Design review of the part built by this model. Coordinates are the model's own, in mm. A direction names the side the tool comes from. Coordinates: 2 decimals unless noted, no trailing zeros. Write each loop counter-clockwise with the first axis right and the second up, starting at its lowest first coordinate (ties: lowest second). Pieces come first, ordered by that corner, then holes.
Q1. Take a section at B-B (z = 0). Give the boundary of the cut face in (x, y), and give its area (3 significant figures).
Q2. For probe 1 along X at (y, z) = (1, 0); probe 2 along X at (y, z) = (-2.5, -5); probe 3 along Y at (x, z) = (6.5, 5.5), list the stretches that pass through material, from the lowest coordinate up.
Q3. Machinability: for faces 1 (the flat face through (-11.9, -1, -23.4)), 2 (the cylindrical face through (25.297, -0.507, -25.359)), 3 (the flat face through (-16, 0, 20)), which of the approach directions +Z, -Z, +X, -X, +Y, -Y give a long, thin tool a straight path to every point of the face, cutting with its end or side? Answer none if there is none.
Q4. Take a section at C-C (y = -23). Give the boundary of the cut face in (x, z).
Q5. Insertion check: pin 1 (6 mm diameter, centred on y = -26.5, z = 6.5, fed in from -X); pin 2 (2 mm diameter, centred on y = -2.5, z = 7, fed in from -X); pin 3 (1.5 mm diameter, centred on x = 4.5, y = -24.5, fed in from +Z). Each pin has a flat end and moves straight along its axis. Give the tip position at first contact, or say it passes through.
Q6. Take a section at A-A (x = 0). Give the boundary of the cut face in (y, z), and give its area (3 significant figures).
Q7. Mouldability with a two-part tool opening along Z and no side actions: class faces 4 (the cylindrical face through (-25.359, -0.507, 25.297)), 5 (the cylindrical face through (-5.47, 0.99, 24.65)), 6 (the flat face through (0, 0, 0)) as pulls with the +Z half, pulls with the -Z half, needs draft (parallel to the pull), parting line crosses it, or undercut.
Q8. Take a section at D-D (x = 20). State how many separate pieces and enclosed holes the cut face has, and give its area (3 significant figures).
```python
from build123d import *

# Parameters (mm, degrees)
SKETCH_1_R          = 25.25
SKETCH_1_R_2        = 23.25
EXTRUDE_1_DEPTH     = 2
SKETCH_2_W          = 53
SKETCH_2_H          = 53
EXTRUDE_1_2_DEPTH   = 1
FILLET_1_R          = 4
SKETCH_3_R          = 22.75
EXTRUDE_2_DEPTH     = 10
SKETCH_5_R          = 2
CUT_EXTRUDE_1_DEPTH = 10


# Read off the part's stored shape, not the designer's step: the loft step
with BuildPart() as part:
    # Sketch 1 → Extrude 1 (new body)
    with BuildSketch(Plane(origin=(0, 0, 0), x_dir=(1, 0, 0), z_dir=(0, 1, 0))):
        Circle(SKETCH_1_R)
        Circle(SKETCH_1_R_2, mode=Mode.SUBTRACT)
    extrude(amount=EXTRUDE_1_DEPTH)

    # Sketch 2 → Extrude 1 2 (add)
    with BuildSketch(Plane.XZ):
        Rectangle(SKETCH_2_W, SKETCH_2_H)
    extrude(amount=EXTRUDE_1_2_DEPTH)

    # Fillet 1
    fillet_1_edges = [part.edges().sort_by_distance(p)[0] for p in [
        (26.5, -0.5, 26.5),
        (-26.5, -0.5, 26.5),
        (-26.5, -0.5, -26.5),
        (26.5, -0.5, -26.5),
    ]]
    fillet(fillet_1_edges, radius=FILLET_1_R)



with BuildPart() as body_2:
    # Sketch 3 → Extrude 2 (new body)
    with BuildSketch(Plane(origin=(0, -30, 0), x_dir=(1, 0, 0), z_dir=(0, 1, 0))):
        with Locations(Location((0, 0, 0), (0, 0, 270))):
            Circle(SKETCH_3_R)
    extrude(amount=EXTRUDE_2_DEPTH)


with BuildPart() as part_1:
    add(part.part)

    add(body_2.part)  # Loft 3 merges body 2
    # Loft 3 outline → Loft 3 (revolve)
    with BuildSketch(Plane.XY):
        Polygon((0, -20), (22.75, -20), (26, -1), (0, -1), align=None)
    revolve(axis=Axis((0, 0, 0), (0, 1, 0)))

    # Sketch 5 → Cut-Extrude 1 (cut)
    with BuildSketch(Plane(origin=(0, 0, 0), x_dir=(1, 0, 0), z_dir=(0, 1, 0))):
        with Locations(Location((-21.213203436, 21.213203436, 0), (0, 0, 270))):
            Circle(SKETCH_5_R)
        with Locations(Location((-21.213203436, -21.213203436, 0), (0, 0, 270))):
            Circle(SKETCH_5_R)
        with Locations(Location((21.213203436, -21.213203436, 0), (0, 0, 270))):
            Circle(SKETCH_5_R)
        with Locations(Location((21.213203436, 21.213203436, 0), (0, 0, 270))):
            Circle(SKETCH_5_R)
    extrude(amount=-CUT_EXTRUDE_1_DEPTH, mode=Mode.SUBTRACT)


solid = part_1.part
```
Response:
1. outline: (-26.5, -1) - (-26, -1) - (-22.75, -20) - (-22.75, -30) - (22.75, -30) - (22.75, -20) - (26, -1) - (26.5, -1) - (26.5, 0) - (25.25, 0) - (25.25, 2) - (23.25, 2) - (23.25, 0) - (-23.25, 0) - (-23.25, 2) - (-25.25, 2) - (-25.25, 0) - (-26.5, 0) - close
1. area: 1,440 mm2
2. probe 1: x = -25.25 to -23.25, 23.25 to 25.25
2. probe 2: x = -25.25 to 25.25
2. probe 3: y = -30 to 0
3. face 1: -Y
3. face 2: -Z, +X, +Y, -Y
3. face 3: +Y
4. outline: circle Ø45.5 at (0, 0)
5. pin 1: stops at x = -22.48
5. pin 2: stops at x = -25.09
5. pin 3: stops at z = 22.44
6. outline: (-30, -22.75) - (-20, -22.75) - (-1, -26) - (-1, -26.5) - (0, -26.5) - (0, -25.25) - (2, -25.25) - (2, -23.25) - (0, -23.25) - (0, 23.25) - (2, 23.25) - (2, 25.25) - (0, 25.25) - (0, 26.5) - (-1, 26.5) - (-1, 26) - (-20, 22.75) - (-30, 22.75) - close
6. area: 1,440 mm2
7. face 4: pulls with the +Z half
7. face 5: parting line crosses it
7. face 6: undercut
8. separate pieces: 3
8. enclosed holes: 0
8. area: 805 mm2
